Solid Edge part; units mm, degrees
sketch "Sketch1" plane through (0, 0, 0) normal (0, 0, 1) x (1, 0, 0)
  line L0 (0, 0) -> (16.3011, 0)
  line L1 (16.3011, 1) -> (16.3011, 0)
  line L2 (16.3011, 1) -> (0, 1)
  line L3 (0, 1) -> (0, 0)
extrude "Protrusion1" add sketch "Sketch1" along normal blind 7
sketch "Sketch2" plane through (0, 0, 0) normal (0, 0, 1) x (1, 0, 0)
  line L0 (0, 0) -> (0, -1)
  line L1 (0, -1) -> (16.3011, -1)
  line L2 (16.3011, -1) -> (16.3011, 0)
  line L3 (16.3011, 1) -> (16.3011, 0)
  line L4 (16.3011, 1) -> (0, 1)
  line L5 (0, 1) -> (0, 0)
extrude "ProtrusioneEstrusa_6" add sketch "Sketch2" against normal blind 1
fillet "Rotondo_3" radius 0.5 2 edges at (8.1505, 1, -1) (8.1505, 0, 0)
fillet "Rotondo_5" radius 0.5 1 edges at (8.1505, -1, -1)
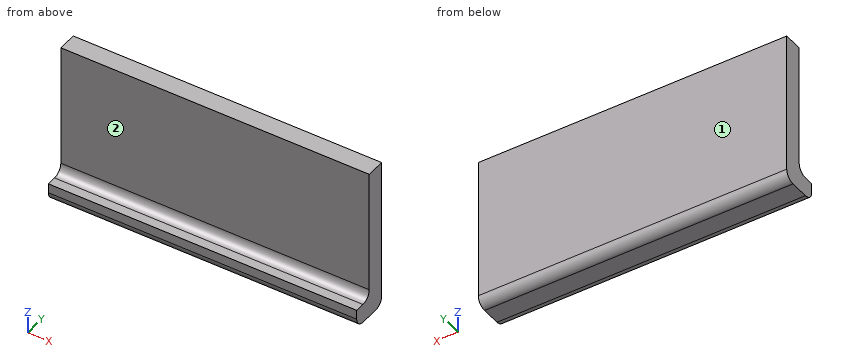
Part model, mm, in its own coordinate system. Face numbers are marked on the shaded views. A direction names the side the tool comes from. Round coordinates to 2 decimals unless told otherwise and drop trailing zeros. Write each loop counter-clockwise with the first axis right and the second up, starting at its lowest first coordinate (ties: lowest second). Pieces come first, ordered by that corner, then holes. Notation, with made-up numbers: M 7.5,60.5 L 18.5,60.5 A24 ccw 18.5,70.5 Z; hole C -20.5,36 d8. An arc over 180 degrees is marked long. Answer as CSV lines item,"result". Start each with the question number.
1) Drop flat-ended pins along their axis: pin 1 (3 mm diameter, centred on x = 4, z = 3.5, fed in from -Y); pin 2 (0.6 mm diameter, centred on x = 8.5, y = -0.5, fed in from +Z). Give the stop position or say it passes through.
2) Band-saw the part on C-C (z = 2.25). List the corners of the cut face in (x, y).
3) Which spindle directions (+Z, -Z, +X, -X, +Y, -Y) get a long thin tool onto all of the face, cutting with end or side? Do the marked faces 1 and 2. Say none if no direction does.
4) Band-saw the part on B-B (y = -0.7). List the corners of the cut face in (x, z), then the cut area to 3 significant figures.
5) Band-saw the part on A-A (x = 6.5). List the corners of the cut face in (y, z).
6) Drill centre lines: L1, parallel to Y at x = 15.5, z = 6.5; L2, parallel to Z at x = 5.5, y = 0.55; L3, parallel to Z at x = 15.5, y = -0.25. Where is each one in solid material? Low to high.
Worked out:
1,pin 1,"y = 0"
1,pin 2,"z = 0.1"
2,outline,"M 0,0 L 16.3,0 L 16.3,1 L 0,1 Z"
3,face 1,"+Z, -Z, +X, -X, +Y"
3,face 2,"+Z, +X, -X, -Y"
4,outline,"M 0,-0.96 L 16.3,-0.96 L 16.3,0 L 0,0 Z"
4,area,"15.6 mm²"
5,outline,"M -1,-0.5 A0.5 ccw -0.5,-1 L 0.5,-1 A0.5 ccw 1,-0.5 L 1,7 L 0,7 L 0,0.5 A0.5 cw -0.5,0 L -1,0 Z"
6,L1,"0 to 1"
6,L2,"-1 to 7"
6,L3,"-1 to 0.07"
